For this review, take the finished solid that the model builds, in its own axes (mm). Face numbers are marked on the shaded views. A direction names the side the tool comes from. Give positions to 0.01 mm unless a question says otherwise; leave off trailing zeros. Order: outer loops, then holes, each group sorted by start corner. A loop starts at its lowest first (then second) coordinate and runs counter-clockwise, first axis right, second up. Notation, with made-up numbers: (60, 0) -> (66, 0) arc R26 ccw to (66, 28) -> close; hole circle Ø5 at (16, -2.75). An arc over 180 degrees is marked (long way). Use CSV: the item, a comma, the result in double quotes. Start each with the question number.
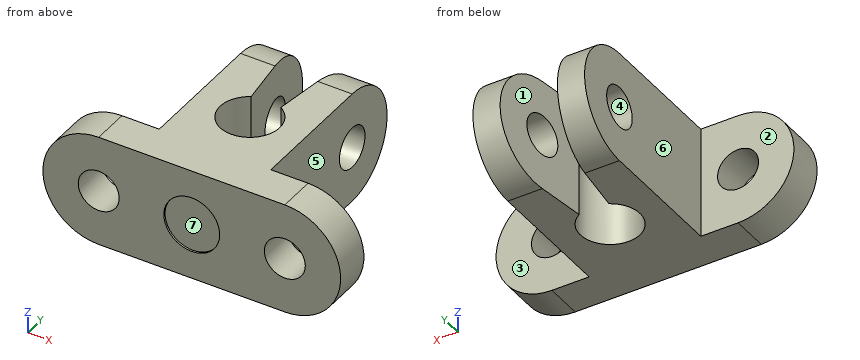
```python
from build123d import *

# Parameters (mm, degrees)
EXTRUDE_1_DEPTH     = 2
SKETCH_2_W          = 6
SKETCH_2_H          = 12
EXTRUDE_2_DEPTH     = 3
FILLET_1_RADIUS     = 3
FILLET_1_LENGTH     = 6
CUT_EXTRUDE_START   = -6
CUT_EXTRUDE_1_DEPTH = 6
SKETCH_4_R          = 1.1
CUT_EXTRUDE_2_DEPTH = 28
SKETCH_7_R          = 1.1
CUT_EXTRUDE_5_DEPTH = 3.5
SKETCH_9_R          = 1.5
CUT_EXTRUDE_7_DEPTH = 0.1


# Read off the part's stored shape, not the designer's step: 切除-拉伸1
with BuildPart() as part:
    # 草图1 → 凸台-拉伸1 (new body)
    with BuildSketch(Plane(origin=(0, 0, 0), x_dir=(1, 0, 0), z_dir=(0, 1, 0))):
        with BuildLine():
            Line((-5, 3), (5, 3))
            ThreePointArc((5, 3), (8, 0), (5, -3))
            Line((5, -3), (-5, -3))
            ThreePointArc((-5, -3), (-8, 0), (-5, 3))
        make_face()
    extrude(amount=EXTRUDE_1_DEPTH)

    # 草图2 → 凸台-拉伸2 (add, symmetric)
    with BuildSketch(Plane(origin=(0, 0, 0), x_dir=(0, 0, -1), z_dir=(1, 0, 0))):
        with Locations((0, 6)):
            Rectangle(SKETCH_2_W, SKETCH_2_H)
    extrude(amount=EXTRUDE_2_DEPTH, both=True)

    # 圆角1: full round fillet: the end face becomes a half cylinder, R = half its width
    fillet_1_face = Plane((0, 12, 0), x_dir=(1, 0, 0), z_dir=(0, 1, 0))  # on the end face: x along it, z out of the body
    fillet_1_slab = fillet_1_face.offset(-FILLET_1_RADIUS / 2) * Box(FILLET_1_LENGTH, 2 * FILLET_1_RADIUS, FILLET_1_RADIUS, mode=Mode.PRIVATE)  # the body's end, R deep
    fillet_1_round = Plane((0, 9, 0), x_dir=(0, 1, 0), z_dir=(1, 0, 0)) * Cylinder(FILLET_1_RADIUS, FILLET_1_LENGTH, mode=Mode.PRIVATE)  # its axis R under the face
    add(fillet_1_slab - fillet_1_round, mode=Mode.SUBTRACT)

    # 切除-拉伸1 outline → 切除-拉伸1 (cut)
    with BuildSketch(Plane(origin=(0, 0, -3), x_dir=(-1, 0, 0), z_dir=(0, 0, -1)).offset(CUT_EXTRUDE_START)):
        with BuildLine():
            ThreePointArc((-0.8, 6.385640646), (0, 3.4), (0.8, 6.385640646))
            Line((0.8, 6.385640646), (1.7488232, 13.59266837))
            Line((1.7488232, 13.59266837), (-1.7488232, 13.59266837))
            Line((-1.7488232, 13.59266837), (-0.8, 6.385640646))
        make_face()
    extrude(amount=CUT_EXTRUDE_1_DEPTH, mode=Mode.SUBTRACT)

    # 草图4 → 切除-拉伸2 (cut)
    with BuildSketch(Plane(origin=(3, 0, 0), x_dir=(0, 0, -1), z_dir=(1, 0, 0))):
        with Locations(Location((0, 9, 0), (0, 0, 270))):
            Circle(SKETCH_4_R)
    extrude(amount=-CUT_EXTRUDE_2_DEPTH, mode=Mode.SUBTRACT)

    # 草图7 → 切除-拉伸5 (cut)
    with BuildSketch(Plane(origin=(0, 2, 0), x_dir=(1, 0, 0), z_dir=(0, 1, 0))):
        with Locations(Location((5, 0, 0), (0, 0, 270))):
            Circle(SKETCH_7_R)
        with Locations(Location((-5, 0, 0), (0, 0, 270))):
            Circle(SKETCH_7_R)
    extrude(amount=-CUT_EXTRUDE_5_DEPTH, mode=Mode.SUBTRACT)

    # 草图9 → 切除-拉伸7 (cut)
    with BuildSketch(Plane.XZ):
        with Locations(Location((0, 0, 0), (0, 0, 270))):
            Circle(SKETCH_9_R)
    extrude(amount=-CUT_EXTRUDE_7_DEPTH, mode=Mode.SUBTRACT)


solid = part.part
```
1. To check wall thickness, follow L1, parallel to X at y = 1, z = 0; L2, parallel to X at y = 0.05, z = 0; L3, parallel to X at y = 3.75, z = 0.55. State the ranges of each line that lie inside material, in increasing order. Write a range as [from, to].
2. Consider section C-C (y = 1.5). State the section outline as (x, z) points.
3. Draft analysis for pull direction X (two halves, no side actions). For the marked faces 4, 5, 6 and 7, state which applies: +X half, -X half, draft (parallel to the pull), parting line (faces both ways), or undercut.
4. Clearance check with flat-ended pins moving along their axes: P1, Ø3.5, axis at y = 9, z = 0, coming from the +X side; P2, Ø3, axis at y = 5.5, z = -1, coming from the -X side; P3, Ø3, axis at x = -5, z = 0, coming from the +Y side. State where each tip first meets the part, or that it passes through.
5. For the marked faces 1, 2 and 3, list the 3-axis set-ups (+Z, -Z, +X, -X, +Y, -Y) from which the entire face can be reached by the end or side of a thin tool; tool diameter is ignored.
6. Consider section B-B (x = -2). State the section outline as (y, z) points.
7. Consider section D-D (z = 0). State how many separate pieces and enclosed holes the cut face has, plus the area to 3 significant figures.
8. Consider section A-A (y = 5). State the section outline as (x, z) points, plus the area to 3 significant figures.
Answer list:
1,L1,"[-8, -6.1], [-3.9, 3.9], [6.1, 8]"
1,L2,"[-8, -6.1], [-3.9, -1.5], [1.5, 3.9], [6.1, 8]"
1,L3,"[-3, -1], [1, 3]"
2,outline,"(-5, -3) -> (5, -3) arc R3 ccw to (5, 3) -> (-5, 3) arc R3 ccw to start; hole circle Ø2.2 at (-5, 0); hole circle Ø2.2 at (5, 0)"
3,face 4,"draft"
3,face 5,"+X half"
3,face 6,"-X half"
3,face 7,"undercut"
4,P1,"x = 3"
4,P2,"x = -3"
4,P3,"y = 2"
5,face 1,"+Z, -Z, +Y"
5,face 2,"+Z, -Z, -X, +Y"
5,face 3,"+Z, -Z, +X, +Y"
6,outline,"(0, -3) -> (9, -3) arc R3 ccw to (9, 3) -> (0, 3) -> close; hole circle Ø2.2 at (9, 0)"
7,separate pieces,"5"
7,enclosed holes,"0"
7,area,"53.8 mm2"
8,outline,"(-3, -3) -> (-1.6, -3) -> (-1.6, 3) -> (-3, 3) -> close; (1.6, -3) -> (3, -3) -> (3, 3) -> (1.6, 3) -> close"
8,area,"16.8 mm2"
